The listing builds one solid part. Answer for the finished solid, in the listing's coordinates (mm). Face numbers are marked on the shaded views. Round coordinates to 2 decimals unless told otherwise and drop trailing zeros. Write each loop counter-clockwise with the first axis right and the second up, starting at its lowest first coordinate (ties: lowest second). Pieces come first, ordered by that corner, then holes.
Item 1: Each of these flat-tipped pins is pushed along its axis until it touches: pin 1 (2 mm diameter, centred on x = 1, y = -2.5, fed in from +Z); pin 2 (1.4 mm diameter, centred on x = -4.2, y = -0.5, fed in from -Z); pin 3 (0.7 mm diameter, centred on x = 7.5, z = 1.5, fed in from -Y); pin 4 (0.7 mm diameter, centred on y = 2.5, z = 1, fed in from -X). Where does it stop, or does it pass through?
Item 2: Find section D-D on x = 3.75. Give the vertices of the cut face in (y, z), then the cut area to 3 significant figures.
Item 3: Find section A-A on y = -0.5. Give the vertices of the cut face in (x, z), then the cut area to 3 significant figures.
Item 4: Find the intervals of material crossed by probe 1 along Y at (x, z) = (4.2, -0.2); probe 2 along X at (y, z) = (-0.05, -0.1); probe 3 along Z at (x, y) = (2.5, 2.3), in increasing order.
Item 5: Find section C-C on z = -0.7. Give the vertices of the cut face in (x, y).
Item 6: For a pull along X with two mould halves and no side action, classify the marked faces 1, 2 and 3 as +X half, -X half, draft (parallel to the pull), parting line (faces both ways), or undercut.
Item 7: Find section B-B on x = 0. Give the vertices of the cut face in (y, z).
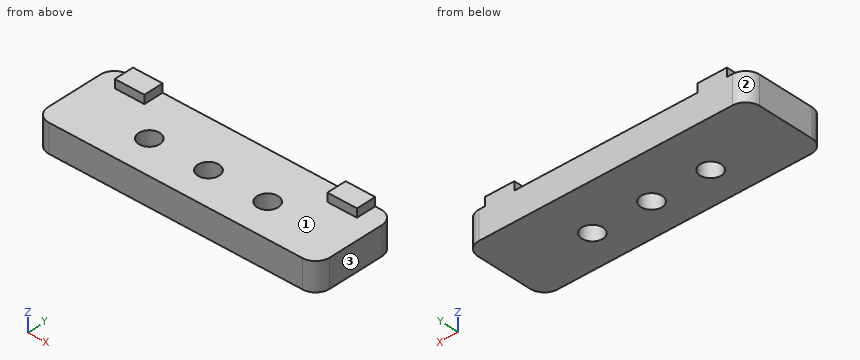
Autodesk Inventor part; units mm, degrees
ref_plane "YZ Plane" through (0, 0, 0) normal (1, 0, 0) x (0, 1, 0)
ref_plane "XZ Plane" through (0, 0, 0) normal (0, 1, 0) x (-1, 0, 0)
ref_plane "XY Plane" through (0, 0, 0) normal (0, 0, 1) x (1, 0, 0)
sketch "Sketch1" plane through (0, 0, 0) normal (0, 0, 1) x (1, 0, 0)
  line L0 (-10, 3) -> (10, 3)
  line L1 (10, 3) -> (10, -3)
  line L2 (10, -3) -> (-10, -3)
  line L3 (-10, -3) -> (-10, 3)
  circle A0 centre (-4.2, -0.5) radius 0.75
  circle A1 centre (4.2, -0.5) radius 0.75
  circle A2 centre (0, -0.5) radius 0.75
  point P0 (0, 0)
  dimension "d0" = 20
  dimension "d1" = 6
  dimension "d2" = 3
  dimension "d3" = 10
  dimension "d7" = 1.5
  dimension "d8" = 1.5
  dimension "d18" = 2.5
  dimension "d19" = 2.5
  dimension "d20" = 1.5
  dimension "d21" = 2.5
  dimension "d22" = 10
  dimension "d23" = 4.2
  dimension "d24" = 4.2
extrude "Extrusion1" add sketch "Sketch1" along normal mid plane 2
sketch "Sketch2" plane through (0, 0, 1) normal (0, 0, 1) x (1, 0, 0)
  line L0 (10, 3) -> (-10, 3)
  line L1 (-8.6, 3) -> (-6.5, 3)
  line L2 (-6.5, 3) -> (-6.5, 1.6)
  line L3 (-6.5, 1.6) -> (-8.6, 1.6)
  line L4 (-8.6, 1.6) -> (-8.6, 3)
  line L5 (6.5, 3) -> (8.6, 3)
  line L6 (8.6, 3) -> (8.6, 1.6)
  line L7 (8.6, 1.6) -> (6.5, 1.6)
  line L8 (6.5, 1.6) -> (6.5, 3)
  line L9 (-10, 3) -> (-10, -3)
  line L10 (10, -3) -> (10, 3)
  point P0 (0, 0)
  point P1 (-6.5, 2.3)
  dimension "d17" = 1.4
  dimension "d30" = 2.1
  dimension "d31" = 6.5
  dimension "d32" = 6.5
  dimension "d33" = 2.1
extrude "Extrusion2" add sketch "Sketch2" along normal blind 0.6
fillet "Fillet1" radius 1 4 edges at (10, 3, 0) (10, -3, 0) (-10, -3, 0) (-10, 3, 0)
equation "\"d7\" = d20"
equation "\"d8\" = d20"
equation "\"d19\" = d18"
equation "\"d21\" = d19"
equation "\"d22\" = d3"
equation "\"d24\" = d23"
equation "\"d33\" = d30"
properties part number "charger_holder_3DPrint"
Check values:
1. pin 1: stops at z = 1
1. pin 2: passes through
1. pin 3: stops at y = 1.6
1. pin 4: stops at x = -9.99
2. outline: (-3, -1) - (-1.1, -1) - (-1.1, 1) - (-3, 1) - close; (0.1, -1) - (3, -1) - (3, 1) - (0.1, 1) - close
2. area: 9.60 mm2
3. outline: (-10, -1) - (-4.95, -1) - (-4.95, 1) - (-10, 1) - close; (-3.45, -1) - (-0.75, -1) - (-0.75, 1) - (-3.45, 1) - close; (0.75, -1) - (3.45, -1) - (3.45, 1) - (0.75, 1) - close; (4.95, -1) - (10, -1) - (10, 1) - (4.95, 1) - close
3. area: 31.0 mm2
4. probe 1: y = -3 to -1.25, 0.25 to 3
4. probe 2: x = -10 to -4.8, -3.6 to -0.6, 0.6 to 3.6, 4.8 to 10
4. probe 3: z = -1 to 1
5. outline: (-10, -2) arc R1 ccw to (-9, -3) - (9, -3) arc R1 ccw to (10, -2) - (10, 2) arc R1 ccw to (9, 3) - (-9, 3) arc R1 ccw to (-10, 2) - close; hole circle Ø1.5 at (-4.2, -0.5); hole circle Ø1.5 at (0, -0.5); hole circle Ø1.5 at (4.2, -0.5)
6. face 1: undercut
6. face 2: -X half
6. face 3: +X half
7. outline: (-3, -1) - (-1.25, -1) - (-1.25, 1) - (-3, 1) - close; (0.25, -1) - (3, -1) - (3, 1) - (0.25, 1) - close
